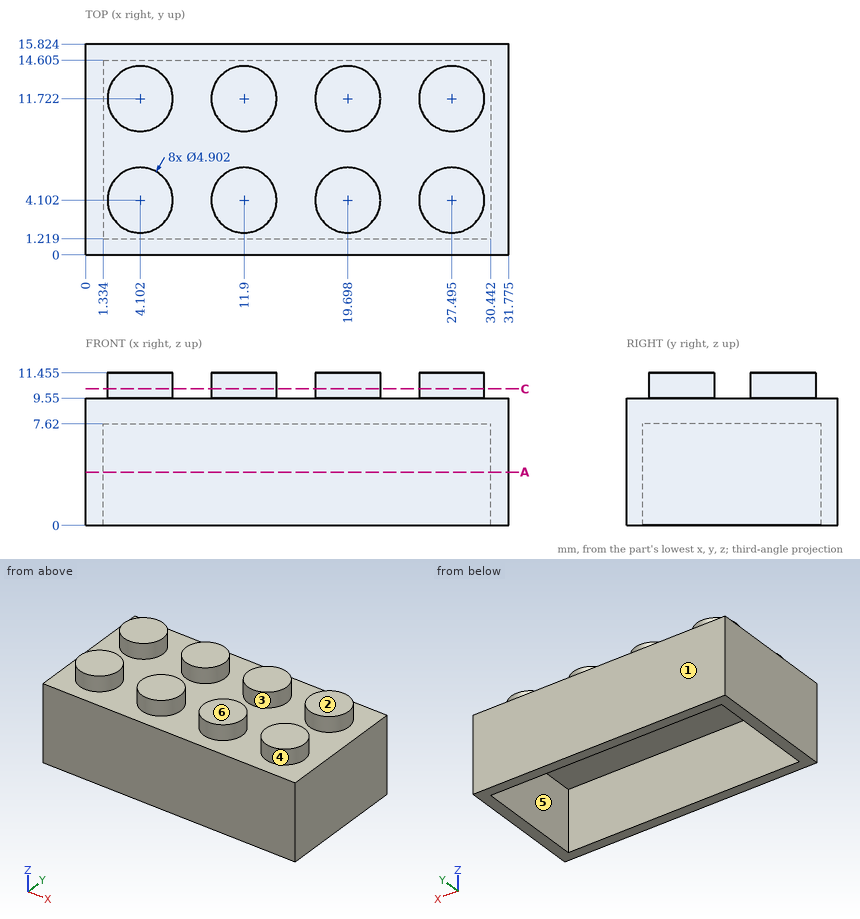
Print and shaded views of the part. All mm, measured from the part's lowest x, y and z. A direction names the side the tool comes from. Coordinates: 2 decimals unless noted, no trailing zeros. Write each loop counter-clockwise with the first axis right and the second up, starting at its lowest first coordinate (ties: lowest second). Pieces come first, ordered by that corner, then holes. Notation, with made-up numbers: (46.5, 24) - (67.5, 24) arc R21 ccw to (67.5, 46) - close; hole circle Ø5 at (43.25, 60.25). An arc over 180 degrees is marked (long way). One line per question, with ' | ' between items. Start each with the question number.
Q1. Pull direction Y, two halves, no side cores. Call the marked faces 1, 2 and 3: pulls with the +Y half, pulls with the -Y half, needs draft (parallel to the pull), parting line crosses it, or undercut.
Q2. Pin check, flat tip, straight feed: pin 1 (3 mm diameter, centred on x = 3.5, y = 10.5, fed in from -Z). Stop position of the tip, or through.
Q3. Cut at C-C, the plane z = 10.25. Give the number of separate pieces and of enclosed holes in the cut face, then the cut area to 3 significant figures.
Q4. 3-axis set-ups, long thin cutter, end or side, ignore diameter. For the marked faces 4, 5 and 6: which of +Z, -Z, +X, -X, +Y, -Y reach the whole face in a straight line?
Q5. Drill centre lines: line 1 (Y direction, x = 20, z = 1.25) (1 decimal); line 2 (X direction, y = 9.5, z = 5) (1 decimal); line 3 (Z direction, x = 19, y = 11.25) (1 decimal). Where is each one in solid material? Low to high. Write a range as [from, to].
Q6. Cut at A-A, the plane z = 4. List the corners of the cut face in (x, y) (1 decimal), then the cut area to 3 significant figures.
Answer below:
1) face 1: pulls with the +Y half | face 2: needs draft | face 3: undercut
2) pin 1: z = 7.62
3) separate pieces: 8 | enclosed holes: 0 | area: 151 mm^2
4) face 4: +Z | face 5: -Z | face 6: +Z, +X, -X, +Y, -Y
5) line 1: [0, 1.2], [14.6, 15.8] | line 2: [0, 1.3], [30.4, 31.8] | line 3: [7.6, 11.5]
6) outline: (0, 0) - (31.8, 0) - (31.8, 15.8) - (0, 15.8) - close; hole (1.3, 1.2) - (30.4, 1.2) - (30.4, 14.6) - (1.3, 14.6) - close | area: 113 mm^2
